CAD build for the part. Positions are in the model's coordinates, mm. A direction names the side the tool comes from. Round coordinates to 2 decimals unless told otherwise and drop trailing zeros. Write each loop counter-clockwise with the first axis right and the second up, starting at its lowest first coordinate (ties: lowest second). Pieces come first, ordered by that corner, then holes. Notation, with made-up numbers: (42, 65.25) -> (50, 65.25) arc R19 cw to (50, 70.25) -> close; hole circle Ø7 at (15.25, 50). An arc over 180 degrees is marked (long way). Put each result on its own line as item: value. Start each with the question number.
1. Saw through at B-B on y = 0. List the corners of the cut face in (x, z), and give its area (3 significant figures).
2. Drill centre lines: line 1 (Y direction, x = -35, z = 2.2); line 2 (Y direction, x = 27, z = 1.4); line 3 (X direction, y = -8.5, z = -8). Where is each one in solid material? Low to high. Write a range as from..to.
3. Saw through at D-D on y = -14.5. List the corners of the cut face in (x, z), and give its area (3 significant figures).
4. Pull direction Y, two halves, no side cores. Call faces 1 (the flat face through (27, 13, 1)), 2 (the flat face through (40, 0, 1)), 3 (the cylindrical face through (28.5, -0.07, 1.48)), 4 (the cylindrical face through (36.2, 8.9, 1.5)): pulls with the +Y half, pulls with the -Y half, needs draft (parallel to the pull), parting line crosses it, or undercut.
5. Flat gauge pins, fed straight in: P1, Ø1.5, axis at x = -17.5, z = -16.5, coming from the +Y side; P2, Ø12.5, axis at x = -23.5, y = -6.5, coming from the -Z side; P3, Ø4, axis at x = -35, y = 0, coming from the -Z side; P4, Ø0.9, axis at x = -31.5, z = 1.5, coming from the -Y side. Where does each tip first touch, or does it go through?
6. Saw through at C-C on x = 35. List the corners of the cut face in (y, z), and give its area (3 significant figures).
7. 3-axis set-ups, long thin cutter, end or side, ignore diameter. For faces 5 (the cylindrical face through (-2.62, 19.93, -8.83)), 6 (the flat face through (27, -13, 1)), 7 (the flat face through (-28, 13, 1)): which of +Z, -Z, +X, -X, +Y, -Y reach the whole face in a straight line?
8. Saw through at A-A on x = 0. List the corners of the cut face in (y, z), and give its area (3 significant figures).
from build123d import *

# Parameters (mm, degrees)
SKETCH_1_W          = 80
SKETCH_1_H          = 26
SKETCH_1_R          = 1.5
EXTRUDE_1_DEPTH     = 3
SKETCH_2_R          = 20.1
EXTRUDE_2_DEPTH     = 24
SKETCH_3_R          = 18.7
CUT_EXTRUDE_1_DEPTH = 25


with BuildPart() as part:
    # 草图1 → 凸台-拉伸1 (new body)
    with BuildSketch(Plane.XY):
        Rectangle(SKETCH_1_W, SKETCH_1_H)
        with Locations((-35, 0)):
            Circle(SKETCH_1_R, mode=Mode.SUBTRACT)
        with Locations((-27, 0)):
            Circle(SKETCH_1_R, mode=Mode.SUBTRACT)
        with Locations((-35, 8)):
            Circle(SKETCH_1_R, mode=Mode.SUBTRACT)
        with Locations((-35, -8)):
            Circle(SKETCH_1_R, mode=Mode.SUBTRACT)
        with Locations(Location((35, -8, 0), (0, 0, 180))):
            Circle(SKETCH_1_R, mode=Mode.SUBTRACT)
        with Locations(Location((35, 8, 0), (0, 0, 180))):
            Circle(SKETCH_1_R, mode=Mode.SUBTRACT)
        with Locations(Location((35, 0, 0), (0, 0, 180))):
            Circle(SKETCH_1_R, mode=Mode.SUBTRACT)
        with Locations(Location((27, 0, 0), (0, 0, 180))):
            Circle(SKETCH_1_R, mode=Mode.SUBTRACT)
    extrude(amount=EXTRUDE_1_DEPTH)

    # 草图2 → 凸台-拉伸2 (add)
    with BuildSketch(Plane.XY.offset(3)):
        Circle(SKETCH_2_R)
    extrude(amount=-EXTRUDE_2_DEPTH)

    # 草图3 → 切除-拉伸1 (cut)
    with BuildSketch(Plane(origin=(0, 0, -21), x_dir=(-1, 0, 0), z_dir=(0, 0, -1))):
        Circle(SKETCH_3_R)
    extrude(amount=-CUT_EXTRUDE_1_DEPTH, mode=Mode.SUBTRACT)


solid = part.part
Return value:
1. outline: (-40, 0) -> (-36.5, 0) -> (-36.5, 3) -> (-40, 3) -> close; (-33.5, 0) -> (-28.5, 0) -> (-28.5, 3) -> (-33.5, 3) -> close; (-25.5, 0) -> (-20.1, 0) -> (-20.1, -21) -> (-18.7, -21) -> (-18.7, 3) -> (-25.5, 3) -> close; (18.7, -21) -> (20.1, -21) -> (20.1, 0) -> (25.5, 0) -> (25.5, 3) -> (18.7, 3) -> close; (28.5, 0) -> (33.5, 0) -> (33.5, 3) -> (28.5, 3) -> close; (36.5, 0) -> (40, 0) -> (40, 3) -> (36.5, 3) -> close
1. area: 151 mm^2
2. line 1: y = -13..-9.5, -6.5..-1.5, 1.5..6.5, 9.5..13
2. line 2: y = -13..-1.5, 1.5..13
2. line 3: x = -18.21..-16.66, 16.66..18.21
3. outline: (-13.92, -21) -> (-11.81, -21) -> (-11.81, 3) -> (-13.92, 3) -> close; (11.81, -21) -> (13.92, -21) -> (13.92, 3) -> (11.81, 3) -> close
3. area: 101 mm^2
4. face 1: pulls with the +Y half
4. face 2: needs draft
4. face 3: undercut
4. face 4: undercut
5. P1: stops at y = 11.11
5. P2: stops at z = -21
5. P3: stops at z = 0
5. P4: stops at y = -13
6. outline: (-13, 0) -> (-9.5, 0) -> (-9.5, 3) -> (-13, 3) -> close; (-6.5, 0) -> (-1.5, 0) -> (-1.5, 3) -> (-6.5, 3) -> close; (1.5, 0) -> (6.5, 0) -> (6.5, 3) -> (1.5, 3) -> close; (9.5, 0) -> (13, 0) -> (13, 3) -> (9.5, 3) -> close
6. area: 51.0 mm^2
7. face 5: -Z
7. face 6: +Z, -Z, +X, -Y
7. face 7: +Z, -Z, -X, +Y
8. outline: (-20.1, -21) -> (-18.7, -21) -> (-18.7, 3) -> (-20.1, 3) -> close; (18.7, -21) -> (20.1, -21) -> (20.1, 3) -> (18.7, 3) -> close
8. area: 67.2 mm^2
